The figure shows three views and two pictorial views of one solid part (mm, origin at its lowest corner). Answer the questions. Round coordinates to 2 decimals unless told otherwise and drop trailing zeros. Order: outer loops, then holes, each group sorted by start corner. A loop starts at its lowest first (then second) coordinate and runs counter-clockwise, first axis right, second up. Notation, with made-up numbers: (77.25, 83.5) -> (95.25, 83.5) arc R17 cw to (95.25, 115.5) -> close; hole circle Ø2 at (69, 46.25). An arc over 180 degrees is marked (long way). Return JSON: item names as keys, results as strings. Group by question number.
(1) Each of these flat-tipped pins is pushed along its axis until it touches: pin 1 (6 mm diameter, centred on y = 37, z = 2.5, fed in from -X); pin 2 (1 mm diameter, centred on x = 12.5, z = 11.5, fed in from -Y); pin 3 (5 mm diameter, centred on y = 7.5, z = 16.5, fed in from -X) (1 decimal); pin 4 (8 mm diameter, centred on x = 22, y = 12.5, fed in from -Z). Where does it stop, or does it pass through?
(2) The part is cut by section A-A (y = 25.37). Determine the outline of the cut face in (x, z), plus the area to 3 significant figures.
(3) Consider line 1 (Y direction, x = 25.37, z = 10); line 2 (X direction, y = 25.5, z = 20); line 3 (Y direction, x = 3, z = 9.25). Determine where each line is inside the solid, lowest interval first. Write a range as [from, to].
(4) The part is cut by section C-C (z = 15.25). Determine the outline of the cut face in (x, y), plus the area to 3 significant figures.
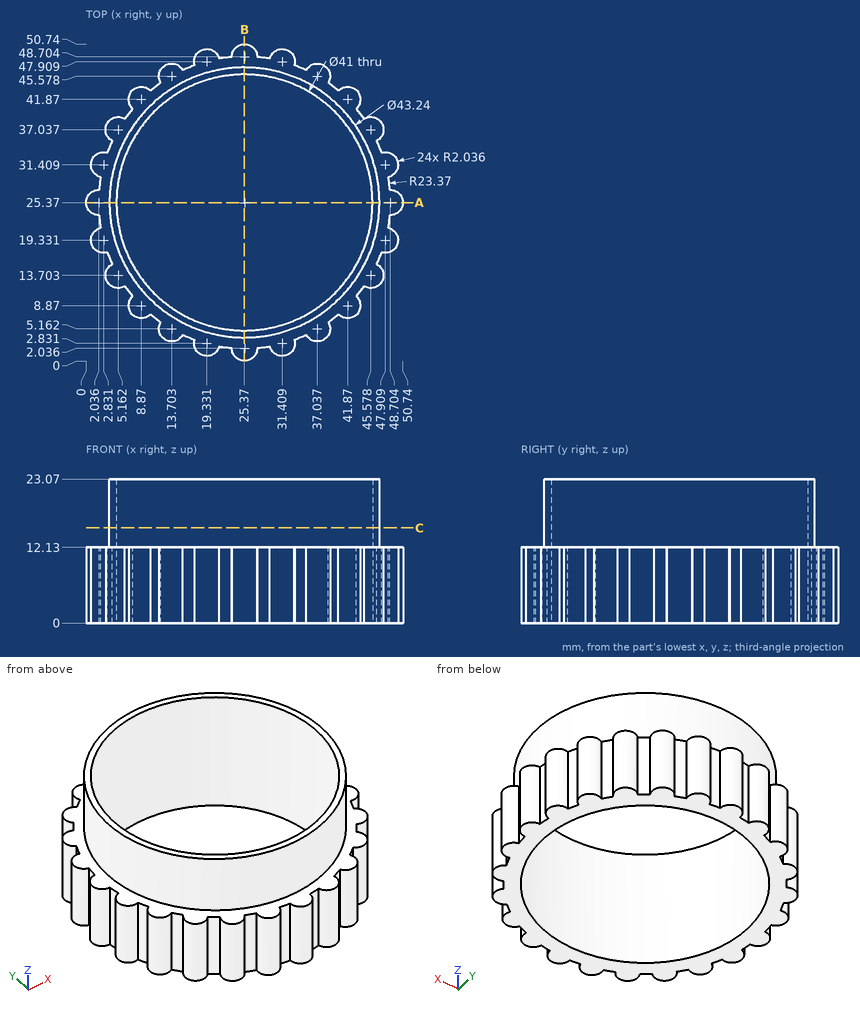
Answer below:
{
 "1": {"pin 1": "stops at x = 3.13", "pin 2": "stops at y = 3.25", "pin 3": "stops at x = 10.2", "pin 4": "passes through"},
 "2": {"outline": "(0, 0) -> (4.87, 0) -> (4.87, 23.07) -> (3.75, 23.07) -> (3.75, 12.13) -> (0, 12.13) -> close; (45.87, 0) -> (50.74, 0) -> (50.74, 12.13) -> (46.99, 12.13) -> (46.99, 23.07) -> (45.87, 23.07) -> close", "area": "143 mm²"},
 "3": {"line 1": "y = [0, 4.87], [45.87, 50.74]", "line 2": "x = [3.75, 4.87], [45.87, 46.99]", "line 3": "y = [17.3, 33.44]"},
 "4": {"outline": "circle Ø43.24 at (25.37, 25.37); hole circle Ø41 at (25.37, 25.37)", "area": "148 mm²"}
}
